Build history of the part. All positions in model axes, mm. Face numbers are marked on the shaded views. A direction names the side the tool comes from. Round coordinates to 2 decimals unless told otherwise and drop trailing zeros. Write each loop counter-clockwise with the first axis right and the second up, starting at its lowest first coordinate (ties: lowest second). Pieces come first, ordered by that corner, then holes. Notation, with made-up numbers: (-36.75, 68.5) -> (-31.75, 68.5) arc R11 cw to (-31.75, 88.5) -> close; hole circle Ø8 at (80, 51). An arc over 180 degrees is marked (long way). Answer in a Markdown table with one row per item.
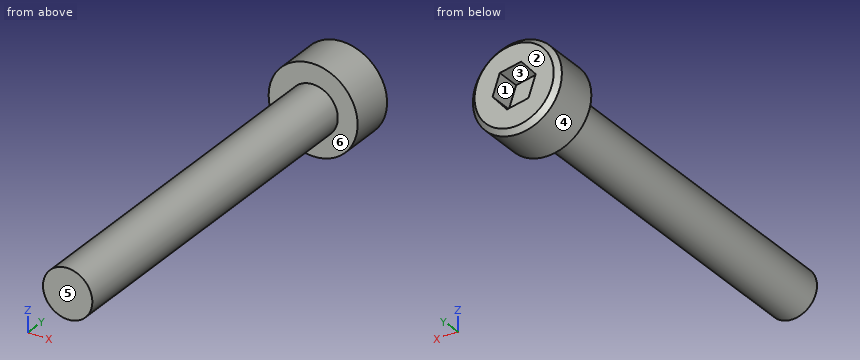
Autodesk Inventor part; units mm, degrees
ref_plane "YZ Plane" through (0, 0, 0) normal (1, 0, 0) x (0, 1, 0)
ref_plane "XZ Plane" through (0, 0, 0) normal (0, 1, 0) x (-1, 0, 0)
ref_plane "XY Plane" through (0, 0, 0) normal (0, 0, 1) x (1, 0, 0)
sketch "Sketch1" plane through (0, 0, 0) normal (0, 0, 1) x (1, 0, 0)
  line L0 (-9.9228, -25) -> (-13.5328, -25)
  line L1 (-13.5328, -25) -> (-13.5328, -21)
  line L2 (-13.5328, -21) -> (-9.9228, -21)
  line L3 (-9.9228, -21) -> (-9.9228, -25)
  line L4 (-9.9228, -25) -> (-9.9228, -55)
  line L5 (-9.9228, -55) -> (-11.9228, -55)
  line L6 (-11.9228, -55) -> (-11.9228, -25)
  point P0 (0, 0)
  dimension "d0" = 3.61
  dimension "d1" = 4
  dimension "d3" = 2
  dimension "d16" = 30
revolve "Revolution1" add sketch "Sketch1" angle 360 about axis through (-9.9228, -25, 0) along (0, -1, 0)
chamfer "Chamfer1" distance 0.4 angle 45 1 edges at (-6.3128, -21, 0)
sketch "Boceto2" plane through (-9.9228, -21, 0) normal (0, 1, 0) x (1, 0, 0)
  line L0 (1.1641, -1.3443) -> (-0.5821, -1.6803)
  line L1 (-0.5821, -1.6803) -> (-1.7462, -0.336)
  line L2 (-1.7462, -0.336) -> (-1.1641, 1.3443)
  line L3 (-1.1641, 1.3443) -> (0.5821, 1.6803)
  line L4 (0.5821, 1.6803) -> (1.7462, 0.336)
  line L5 (1.7462, 0.336) -> (1.1641, -1.3443)
  point P0 (9.9228, 0)
  point P1 (0, 0)
  dimension "d11" = 3.08
extrude "Extrusión1" cut sketch "Boceto2" against normal blind 2
thread "Rosca1"
properties part number "Tornillo Allen cabeza cilindrica M4x30mm"
Q1. Saw through at A-A on y = -51. Write the cut outline in (x, z).
A:
| item | result |
|---|---|
| outline | circle Ø4 at (-9.92, 0) |
Q2. Saw through at B-B on z = 0. Write the cut outline in (x, y).
A:
| item | result |
|---|---|
| outline | (-13.53, -25) -> (-11.92, -25) -> (-11.92, -55) -> (-7.92, -55) -> (-7.92, -25) -> (-6.31, -25) -> (-6.31, -21.4) -> (-6.71, -21) -> (-8.29, -21) -> (-8.29, -23) -> (-11.55, -23) -> (-11.55, -21) -> (-13.13, -21) -> (-13.53, -21.4) -> close |
Q3. Two-plate mould, pull along Z, no slides. Class the marked faces 1, 2, 3 and 4: released by +Z, released by -Z, zero draft, split by the parting line, or undercut.
A:
| item | result |
|---|---|
| face 1 | undercut |
| face 2 | zero draft |
| face 3 | undercut |
| face 4 | split by the parting line |
Q4. Drop flat-ended pins along their axis: P1, Ø1, axis at x = -11.5, y = -38.5, coming from the -Z side; P2, Ø1.7, axis at x = -10, z = 0.5, coming from the +Y side; P3, Ø2, axis at y = -38, z = 2.5, coming from the -X side. Give the stop position or say it passes through.
A:
| item | result |
|---|---|
| P1 | z = -1.69 |
| P2 | y = -23 |
| P3 | x = -11.25 |
Q5. Which spindle directions (+Z, -Z, +X, -X, +Y, -Y) get a long thin tool onto all of the face, cutting with end or side? Do the marked faces 5 and 6. Say none if no direction does.
A:
| item | result |
|---|---|
| face 5 | +Z, -Z, +X, -X, -Y |
| face 6 | -Y |
Q6. Wall check: line 1 (Y direction, x = -10.5, z = -3); line 2 (Y direction, x = -11, z = 0.75); line 3 (X direction, y = -21.5, z = 0.25). Give the ranges that are in metal, low to high. Write a range as [from, to].
A:
| item | result |
|---|---|
| line 1 | [-25, -21] |
| line 2 | [-55, -23] |
| line 3 | [-13.52, -11.64], [-8.38, -6.32] |
